Part print with two shaded views. Sizes in mm from the minimum x, y, z corner. A direction names the side the tool comes from. Coordinates: 2 decimals unless noted, no trailing zeros. Loops run counter-clockwise (first coordinate to the right, second up) from the corner with the lowest first, then second, coordinate; pieces in that order, holes last.
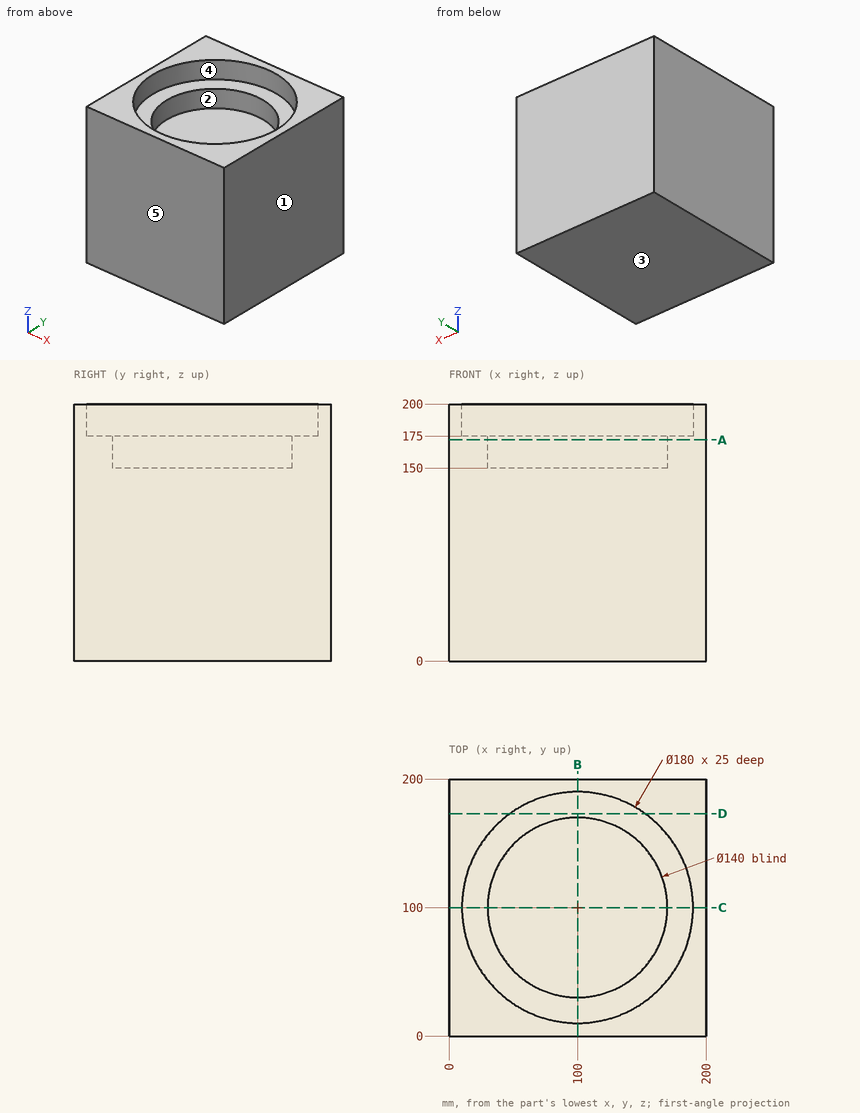
Q1. Slice it at A-A (z = 172). List the corners of the cut face in (x, y), and give its area (3 significant figures).
Answers:
outline: (0, 0) - (200, 0) - (200, 200) - (0, 200) - close; hole circle Ø140 at (100, 100)
area: 24,600 mm2
Q2. Drill centre lines: line 1 (Y direction, x = 100, z = 166); line 2 (Z direction, x = 140.5, y = 107); line 3 (Z direction, x = 122, y = 17). Where is each one in solid material? Low to high.
Answers:
line 1: y = 0 to 30, 170 to 200
line 2: z = 0 to 150
line 3: z = 0 to 175
Q3. Flat gauge pins, fed straight in: P1, Ø5, axis at x = 60.5, y = 171, coming from the +Z side; P2, Ø4, axis at x = 43, y = 94.5, coming from the +Z side; P3, Ø10, axis at x = 57, z = 89, coming from the -Y side. Where does each tip first touch, or does it go through?
Answers:
P1: stops at z = 175
P2: stops at z = 150
P3: stops at y = 0
Q4. Slice it at B-B (x = 100). List the corners of the cut face in (y, z).
Answers:
outline: (0, 0) - (200, 0) - (200, 200) - (190, 200) - (190, 175) - (170, 175) - (170, 150) - (30, 150) - (30, 175) - (10, 175) - (10, 200) - (0, 200) - close
Q5. Mould opens along X. For the marked faces 1, 2 and 3 say: +X half, -X half, draft (parallel to the pull), parting line (faces both ways), or undercut.
Answers:
face 1: +X half
face 2: undercut
face 3: draft
Q6. Slice it at D-D (y = 173). List the corners of the cut face in (x, z), and give its area (3 significant figures).
Answers:
outline: (0, 0) - (200, 0) - (200, 200) - (152.64, 200) - (152.64, 175) - (47.36, 175) - (47.36, 200) - (0, 200) - close
area: 37,400 mm2
Q7. Which spindle directions (+Z, -Z, +X, -X, +Y, -Y) get a long thin tool onto all of the face, cutting with end or side? Do the marked faces 4 and 5. Say none if no direction does.
Answers:
face 4: +Z
face 5: +Z, -Z, +X, -X, -Y
